Build history of the part. All positions in model axes, mm. Face numbers are marked on the shaded views. A direction names the side the tool comes from. Give positions to 0.01 mm unless a question says otherwise; leave off trailing zeros. Order: outer loops, then holes, each group sorted by start corner. A loop starts at its lowest first (then second) coordinate and runs counter-clockwise, first axis right, second up. Notation, with made-up numbers: M -37.5,-3 L 1.5,-3 A27 ccw 1.5,21 Z; hole C -5,65 d4. An arc over 180 degrees is marked long. Answer as CSV lines item,"result".
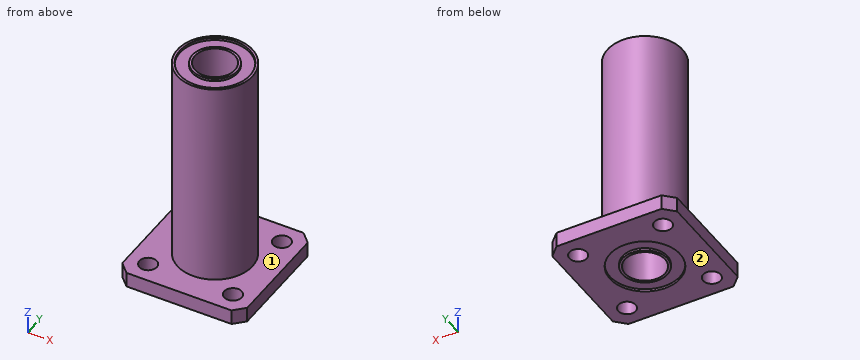
from build123d import *

# Parameters (mm, degrees)
SKETCH_W     = 25
SKETCH_H     = 25
SKETCH_R     = 7.5
SKETCH_R_2   = 1.75
PAD_DEPTH    = 3
SKETCH002_W  = 0.5
SKETCH002_H  = 45
CHAMFER_SIZE = 2


with BuildPart() as part:
    # Sketch → Pad (new body)
    with BuildSketch(Plane.XY):
        Rectangle(SKETCH_W, SKETCH_H)
        Circle(SKETCH_R, mode=Mode.SUBTRACT)
        with Locations((8.485281, 8.485281)):
            Circle(SKETCH_R_2, mode=Mode.SUBTRACT)
        with Locations((-8.485281, 8.485281)):
            Circle(SKETCH_R_2, mode=Mode.SUBTRACT)
        with Locations((8.485281, -8.485281)):
            Circle(SKETCH_R_2, mode=Mode.SUBTRACT)
        with Locations((-8.485281, -8.485281)):
            Circle(SKETCH_R_2, mode=Mode.SUBTRACT)
    extrude(amount=PAD_DEPTH)

    # Sketch001 → Revolution (revolve)
    with BuildSketch(Plane.XZ):
        Polygon((4, 45), (4, 0), (4.5, 0), (4.5, 0.5), (7, 0.5), (7, 44.5), (4.5, 44.5), (4.5, 45), align=None)
    revolve(axis=Axis((0, 0, 0), (0, 0, 1)))

    # Sketch002 → Revolution001 (revolve)
    with BuildSketch(Plane.XZ):
        with Locations((7.25, 22.5)):
            Rectangle(SKETCH002_W, SKETCH002_H)
    revolve(axis=Axis((0, 0, 0), (0, 0, 1)))

    # Chamfer
    chamfer_edges = [part.edges().sort_by_distance(p)[0] for p in [
        (-12.5, -12.5, 1.5),
        (-12.5, 12.5, 1.5),
        (12.5, 12.5, 1.5),
        (12.5, -12.5, 1.5),
    ]]
    chamfer(chamfer_edges, length=CHAMFER_SIZE)


solid = part.part
Item 1: Band-saw the part on A-A (x = 0). Give the cut face in (y, z), and give its area (3 significant figures).
Geometry says:
outline,"M -12.5,0 L -7,0 L -7,0.5 L -4.5,0.5 L -4.5,0 L -4,0 L -4,45 L -4.5,45 L -4.5,44.5 L -7,44.5 L -7,45 L -7.5,45 L -7.5,3 L -12.5,3 Z; M 4,0 L 4.5,0 L 4.5,0.5 L 7,0.5 L 7,0 L 12.5,0 L 12.5,3 L 7.5,3 L 7.5,45 L 7,45 L 7,44.5 L 4.5,44.5 L 4.5,45 L 4,45 Z"
area,"340 mm2"
Item 2: Probe line 1 along Y through (x, z) = (0, 35.5); line 2 along Y through (x, z) = (-3.25, 10.5); line 3 along Y through (x, z) = (6, 32). List the from-to ranges inside material, lowest first. Write a range as from..to.
Geometry says:
line 1,"y = -7.5..-4, 4..7.5"
line 2,"y = -6.76..-2.33, 2.33..6.76"
line 3,"y = -4.5..4.5"
Item 3: Drop flat-ended pins along their axis: pin 1 (4 mm diameter, centred on y = 4.5, z = 24.5, fed in from +X); pin 2 (1 mm diameter, centred on x = 7.5, y = 9.5, fed in from +Z); pin 3 (3 mm diameter, centred on x = -8.49, y = -8.49, fed in from +Z); pin 4 (10 mm diameter, centred on y = -9.5, z = 13.5, fed in from -X). Give the stop position or say it passes through.
Geometry says:
pin 1,"stops at x = 7.07"
pin 2,"stops at z = 3"
pin 3,"passes through"
pin 4,"stops at x = -6"
Item 4: Band-saw the part on C-C (y = -8). Give the cut face in (x, z).
Geometry says:
outline,"M -12.5,0 L -10.17,0 L -10.17,3 L -12.5,3 Z; M -6.8,0 L 6.8,0 L 6.8,3 L -6.8,3 Z; M 10.17,0 L 12.5,0 L 12.5,3 L 10.17,3 Z"
Item 5: Band-saw the part on D-D (z = 8). Give the cut face in (x, y).
Geometry says:
outline,"C 0,0 d15; hole C 0,0 d8"
Item 6: 3-axis set-ups, long thin cutter, end or side, ignore diameter. For the marked faces 1 and 2: which of +Z, -Z, +X, -X, +Y, -Y reach the whole face in a straight line?
Geometry says:
face 1,"+Z"
face 2,"-Z, +X, -X, +Y, -Y"
